```python
from build123d import *

# Parameters (mm, degrees)
CBORE_FOR_M2_5_SHCS1_D           = 2.9
CBORE_FOR_M2_5_SHCS1_CBORE_D     = 5.5
CBORE_FOR_M2_5_SHCS1_CBORE_DEPTH = 2.6


with BuildPart() as part:
    # Sketch1 → Revolve1 (revolve)
    with BuildSketch(Plane(origin=(0, 0, 0), x_dir=(0, 0, -1), z_dir=(1, 0, 0))):
        Polygon((-5.5, 5.697418143), (-5.5, 0), (0, 0), (0, 7.5), (-2.5, 7.5), align=None)
    revolve(axis=Axis((0, 7.5, 0), (0, -1, 0)))

    # CBORE for M2.5 SHCS1 (through all)
    with Locations(Plane(origin=(0, 0, 0), x_dir=(-1, 0, 0), z_dir=(0, -1, 0))):
        with Locations((0, 0)):
            CounterBoreHole(CBORE_FOR_M2_5_SHCS1_D / 2, CBORE_FOR_M2_5_SHCS1_CBORE_D / 2, CBORE_FOR_M2_5_SHCS1_CBORE_DEPTH)


solid = part.part
```
Here's how the part is built. I have some questions about the finished solid (model axes, mm). A direction names the side the tool comes from. Give positions to 0.01 mm unless a question says otherwise; leave off trailing zeros. Loops run counter-clockwise (first coordinate to the right, second up) from the corner with the lowest first, then second, coordinate; pieces in that order, holes last. Notation, with made-up numbers: (35.5, -1.75) -> (64.5, -1.75) arc R26 cw to (64.5, 25.25) -> close; hole circle Ø10 at (50.5, 48.25). An arc over 180 degrees is marked (long way). Use one line per item in the form item = value. Start each with the question number.
1) Imagine slicing it at B-B (z = 0). Please give me the cut outline in (x, y), then the cut area to 3 significant figures.
2) Thinking about a two-plate mould opening in X: for faces 3 (the face through (-1.45, 5.08, -0.06)), 4 (the face through (0, 7.5, -2)), 5 (the face through (-0.81, 7.39, 2.56)), which applies, +X half, -X half, draft (parallel to the pull), parting line (faces both ways), or undercut?
3) Imagine slicing it at C-C (y = 4). Please give me the cut outline in (x, z), then the cut area to 3 significant figures.
4) Imagine slicing it at A-A (x = 0). Please give me the cut outline in (y, z).
5) Which directions (+Z, -Z, +X, -X, +Y, -Y) give clear straight access to the entire face, cutting with the end or side of a thin tool? Please do faces 1 (the face through (-3, 0, 1)), 2 (the face through (-1.2, 2.6, 1.2)).
6) Please list where these lines run through material, in increasing order: line 1 along Z through (x, y) = (0, 1.9); line 2 along Z through (x, y) = (0, 5); line 3 along X through (y, z) = (4.75, 0.25).
7) Imagine slicing it at D-D (y = 1). Please give me the cut outline in (x, z), then the cut area to 3 significant figures.
8) For P1, Ø3.5, axis at x = 0, z = 0, coming from the +Y side; P2, Ø3, axis at y = 2, z = -4.5, coming from the +X side; P3, Ø4, axis at y = 5, z = 2.5, coming from the +X side; P4, Ø1, axis at y = 5, z = -3, coming from the +X side, each with a flat end and sliding along its axis, tell me the tip position at first contact or that it passes through.
Check values:
q1.outline = (-5.5, 0) -> (-2.75, 0) -> (-2.75, 2.6) -> (-1.45, 2.6) -> (-1.45, 7.5) -> (-2.5, 7.5) -> (-5.5, 5.7) -> close; (1.45, 2.6) -> (2.75, 2.6) -> (2.75, 0) -> (5.5, 0) -> (5.5, 5.7) -> (2.5, 7.5) -> (1.45, 7.5) -> close
q1.area = 48.6 mm^2
q2.face_3 = undercut
q2.face_4 = draft
q2.face_5 = parting line
q3.outline = circle Ø11 at (0, 0); hole circle Ø2.9 at (0, 0)
q3.area = 88.4 mm^2
q4.outline = (0, -5.5) -> (5.7, -5.5) -> (7.5, -2.5) -> (7.5, -1.45) -> (2.6, -1.45) -> (2.6, -2.75) -> (0, -2.75) -> close; (0, 2.75) -> (2.6, 2.75) -> (2.6, 1.45) -> (7.5, 1.45) -> (7.5, 2.5) -> (5.7, 5.5) -> (0, 5.5) -> close
q5.face_1 = +Z, -Z, +X, -X, -Y
q5.face_2 = -Y
q6.line_1 = -5.5 to -2.75, 2.75 to 5.5
q6.line_2 = -5.5 to -1.45, 1.45 to 5.5
q6.line_3 = -5.49 to -1.43, 1.43 to 5.49
q7.outline = circle Ø11 at (0, 0); hole circle Ø5.5 at (0, 0)
q7.area = 71.3 mm^2
q8.P1 = 7.5
q8.P2 = 4.61
q8.P3 = 5.48
q8.P4 = 4.9
